Geometry check sheet. Reference: the model listing, model coordinates, mm. A direction names the side the tool comes from. Round coordinates to 2 decimals unless told otherwise and drop trailing zeros. Loops run counter-clockwise (first coordinate to the right, second up) from the corner with the lowest first, then second, coordinate; pieces in that order, holes last. Notation, with made-up numbers: (53.5, 40.5) -> (104.5, 40.5) arc R25 cw to (104.5, 71.5) -> close; hole circle Ø2 at (7, 14). An arc over 180 degrees is marked (long way). Use one line per item in the form item = value.
Autodesk Inventor part; units mm, degrees
ref_plane "YZ Plane" through (0, 0, 0) normal (1, 0, 0) x (0, 1, 0)
ref_plane "XZ Plane" through (0, 0, 0) normal (0, 1, 0) x (-1, 0, 0)
ref_plane "XY Plane" through (0, 0, 0) normal (0, 0, 1) x (1, 0, 0)
sketch "Sketch1" plane through (0, 0, 0) normal (0, 0, 1) x (1, 0, 0)
  circle A0 centre (0, 0) radius 2.75
  circle A1 centre (0, 0) radius 6
  circle A2 centre (0, 0) radius 1
  circle A3 centre (0, 0) radius 2.25
  circle A4 centre (0, 0) radius 3.25
  dimension "d0" = 5.5
  dimension "d1" = 12
  dimension "d2" = 2
  dimension "d5" = 4.5
  dimension "d6" = 6.5
extrude "Extrusion1" add sketch "Sketch1" along normal blind 2 contours A0 | A1 | A3 | A4
extrude "Extrusion2" add sketch "Sketch1" against normal blind 3 contours A0 | A1 | A4
extrude "Extrusion3" add sketch "Sketch1" against normal blind 13 contours A1 | A4
extrude "Extrusion4" add sketch "Sketch1" against normal blind 20 contours A1
properties part number "detector holder"
1. Section check D-D (z = -8.5). Record the boundary of the cut face in (x, y), then the cut area to 3 significant figures.
Return value:
outline = circle Ø12 at (0, 0); hole circle Ø5.5 at (0, 0)
area = 89.3 mm2
2. Tool access check on faces 1 (the cylindrical face through (-0.596, -2.685, -7.93)), 2 (the flat face through (3, -3, -20)). Record the directions out of +Z, -Z, +X, -X, +Y, -Y that give a thin tool (end or side, any length) a straight path to the whole face; none if there is none.
Return value:
face_1 = -Z
face_2 = -Z, +X, -X, +Y, -Y
3. Section check C-C (z = -13.75). Record the boundary of the cut face in (x, y).
Return value:
outline = circle Ø12 at (0, 0); hole circle Ø6.5 at (0, 0)
4. Material ranges on line 1 along Y through (x, z) = (0, -15.75); line 2 along Y through (x, z) = (0, -8); line 3 along X through (y, z) = (-1, -2), recorded low to high.
Return value:
line_1 = -6 to -3.25, 3.25 to 6
line_2 = -6 to -2.75, 2.75 to 6
line_3 = -5.92 to -2.02, 2.02 to 5.92
5. Section check A-A (x = 0). Record the boundary of the cut face in (y, z), then the cut area to 3 significant figures.
Return value:
outline = (-6, -20) -> (-3.25, -20) -> (-3.25, -13) -> (-2.75, -13) -> (-2.75, -3) -> (-2.25, -3) -> (-2.25, 0) -> (-1, 0) -> (-1, 2) -> (-6, 2) -> close; (1, 0) -> (2.25, 0) -> (2.25, -3) -> (2.75, -3) -> (2.75, -13) -> (3.25, -13) -> (3.25, -20) -> (6, -20) -> (6, 2) -> (1, 2) -> close
area = 146 mm2
6. Mould release check, pull along Y, two halves, no side actions. Record for faces 3 (the cylindrical face through (0, 1, 1)), 4 (the flat face through (1.2, 0.1, 2)), 5 (the cylindrical face through (-6, 0, -9)), 6 (the cylindrical face through (-0.29, 2.23, -1.48)): released by +Y, released by -Y, zero draft, split by the parting line, or undercut.
Return value:
face_3 = undercut
face_4 = zero draft
face_5 = split by the parting line
face_6 = undercut
7. Gauge pin test, flat ends, axial feed: pin 1 (5 mm diameter, centred on x = 0.5, y = 0.5, fed in from -Z); pin 2 (1.6 mm diameter, centred on x = 0, y = 0, fed in from +Z); pin 3 (2 mm diameter, centred on y = -4.5, z = -15.5, fed in from +X); pin 4 (1 mm diameter, centred on x = -1.5, z = -12.5, fed in from -Y). Record the tip position at first contact, or that the pin passes through.
Return value:
pin_1 = -13
pin_2 = through
pin_3 = 4.87
pin_4 = -5.92
